Input: part model. Units: mm. Frame: model coordinates. A direction names the side the tool comes from. Give positions to 0.01 mm unless a question says otherwise; leave off trailing zeros. Loops run counter-clockwise (first coordinate to the right, second up) from the corner with the lowest first, then second, coordinate; pieces in that order, holes last. Notation, with made-up numbers: (-12.75, 21.5) - (38.25, 21.5) arc R21 cw to (38.25, 48.5) - close; hole circle Ø2 at (88, 61). An arc over 180 degrees is marked (long way). Answer as a JSON object with one key per item and string values.
from build123d import *

# Parameters (mm, degrees)
F3_DEPTH = 19.05
F1_R     = 12.7
F4_DEPTH = 19.05
F2_W     = 127
F2_H     = 101.6
F2_H_2   = 260.35
F5_DEPTH = 19.05


with BuildPart() as f3:
    # F0 (on Front) → F3 (new body)
    with BuildSketch(Plane.XZ):
        Polygon((-678.356835, -30.721705), (-678.356835, -186.296705), (708.359913, -186.296705), (708.359913, 4.203295), (437.832026, 74.053295), (-273.367974, 74.053295), align=None)
    extrude(amount=F3_DEPTH)

    # F1 (on face) → F4 (join)
    with BuildSketch(Plane.XZ):
        with BuildLine():
            Line((-425.853448, 34.603653), (-298.853448, 67.459927))
            Line((-298.853448, 67.459927), (-298.853448, 194.703295))
            ThreePointArc((-298.853448, 194.703295), (-386.76919, 174.422972), (-425.853448, 93.103295))
            Line((-425.853448, 93.103295), (-425.853448, 34.603653))
        make_face()
        with Locations((-362.353448, 143.903295)):
            Circle(F1_R, mode=Mode.SUBTRACT)
        Polygon((-425.853448, -186.296705), (-298.853448, -186.296705), (-298.853448, 67.459927), (-425.853448, 34.603653), align=None)
    extrude(amount=-F4_DEPTH)

    # F2 (on face) → F5 (join)
    with BuildSketch(Plane.XZ):
        with Locations((374.332026, 124.853295)):
            Rectangle(F2_W, F2_H)
        with Locations((374.332026, -56.121705)):
            Rectangle(F2_W, F2_H_2)
    extrude(amount=-F5_DEPTH)


solid = f3.part
Item 1: Contact query for flat-ended pins moving along their axis: P1, Ø10, axis at y = 0, z = 85, coming from the -X side; P2, Ø21, axis at x = 384, y = 7, coming from the +Z side; P3, Ø6, axis at y = 9.5, z = 117.5, coming from the +X side; P4, Ø23, axis at x = -362.35, z = 143.9, coming from the +Y side. Output: stop coordinate, or through.
Geometry check:
{"P1": "stops at x = -425.85", "P2": "stops at z = 175.65", "P3": "stops at x = 437.83", "P4": "passes through"}
Item 2: Cut plane C-C (z = 55). Return loops of the section in (x, y), then the cut area to 3 significant figures.
Geometry check:
{"outline": "(-425.85, 0) - (-347.02, 0) - (-347.02, -19.05) - (511.63, -19.05) - (511.63, 0) - (437.83, 0) - (437.83, 19.05) - (310.83, 19.05) - (310.83, 0) - (-298.85, 0) - (-298.85, 19.05) - (-425.85, 19.05) - close", "area": "21,200 mm2"}
Item 3: Cut plane B-B (x = -320). Return loops of the section in (y, z).
Geometry check:
{"outline": "(-19.05, -186.3) - (19.05, -186.3) - (19.05, 197.23) - (0, 197.23) - (0, 61.99) - (-19.05, 61.99) - close"}
Item 4: Cut plane A-A (y = 12.5). Return loops of the section in (x, z).
Geometry check:
{"outline": "(-425.85, -186.3) - (-298.85, -186.3) - (-298.85, 194.7) arc R104.14 ccw to (-425.85, 93.1) - close; (310.83, -186.3) - (437.83, -186.3) - (437.83, 175.65) - (310.83, 175.65) - close; hole circle Ø25.4 at (-362.35, 143.9)"}
Item 5: Access query for faces 1 (the face through (-554, 0, -99)), 2 (the face through (373, 0, 126)), 3 (the face through (5, -19.05, -54)), 4 (the face through (-363, 19.05, 8)), 5 (the face through (-363, 0, 117)). Directions: +Z, -Z, +X, -X, +Y, -Y. A direction counts if a zero-diameter tool reaches every point of the face in a straight line with its end or side. Return the directions, or none.
Geometry check:
{"face 1": "+Z, -Z, -X, +Y", "face 2": "+Z, +X, -X, -Y", "face 3": "+Z, -Z, +X, -X, -Y", "face 4": "+Z, -Z, +X, -X, +Y", "face 5": "+Z, -X, -Y"}
Item 6: Material intervals for line 1 (X direction, y = 7, z = -116.5); line 2 (Z direction, x = 410, y = 4.5); line 3 (Y direction, x = -484.5, z = -28), sorted ascending. Write a range as [from, to].
Geometry check:
{"line 1": "x = [-425.85, -298.85], [310.83, 437.83]", "line 2": "z = [-186.3, 175.65]", "line 3": "y = [-19.05, 0]"}
Item 7: Cut plane D-D (x = -83.5). Return loops of the section in (y, z).
Geometry check:
{"outline": "(-19.05, -186.3) - (0, -186.3) - (0, 74.05) - (-19.05, 74.05) - close"}
Item 8: Mould query, pull axis X, two halves, no side actions, for faces 6 (the face through (571, 0, -83)), 7 (the face through (2, 0, -54)), 8 (the face through (574.99, -9.39, 38.64)). Classes: released by +X, released by -X, zero draft, split by the parting line, or undercut.
Geometry check:
{"face 6": "zero draft", "face 7": "undercut", "face 8": "released by +X"}
